The figure shows three views and two pictorial views of one solid part (mm, origin at its lowest corner). Answer the questions. A direction names the side the tool comes from. Coordinates: 2 decimals unless noted, no trailing zeros. Loops run counter-clockwise (first coordinate to the right, second up) from the corner with the lowest first, then second, coordinate; pieces in that order, holes last. Notation, with made-up numbers: M 2,67 L 59,67 A8 cw 59,76 Z; hole C -16.5,69 d9. An arc over 180 degrees is marked long. One line per item, written item: value. Start each with the question number.
1. The part is cut by section B-B (y = 2.54). Write down the section's boundary in (x, z), then the cut area to 3 significant figures.
2. The part is cut by section A-A (y = 4.75). Write down the section's boundary in (x, z).
3. A flat-ended cylindrical pin translates along its axis: pin 1 (3 mm diameter, centred on x = 8, z = 4, fed in from -Y). Find the tip coordinate at first contact, or state that the pin passes through.
4. For the marked faces 1 and 2, determine the directions among +Z, -Z, +X, -X, +Y, -Y from which every point of the face is accessible in a straight line to the end or side of a thin tool.
5. Consider probe 1 along X at (y, z) = (3.75, 9.25); probe 2 along Y at (x, z) = (1.3, 5.08); probe 3 along Y at (x, z) = (19.75, 3.25). Determine where each line is inside the solid, lowest interval first.
6. Determine the mould class of the marked faces 3, 4 and 5 for opening direction X: +X half, -X half, draft (parallel to the pull), parting line (faces both ways), or undercut.
7. The part is cut by section D-D (x = 12.7). Write down the section's boundary in (y, z), then the cut area to 3 significant figures.
8. The part is cut by section C-C (z = 5.08). Write down the section's boundary in (x, y).
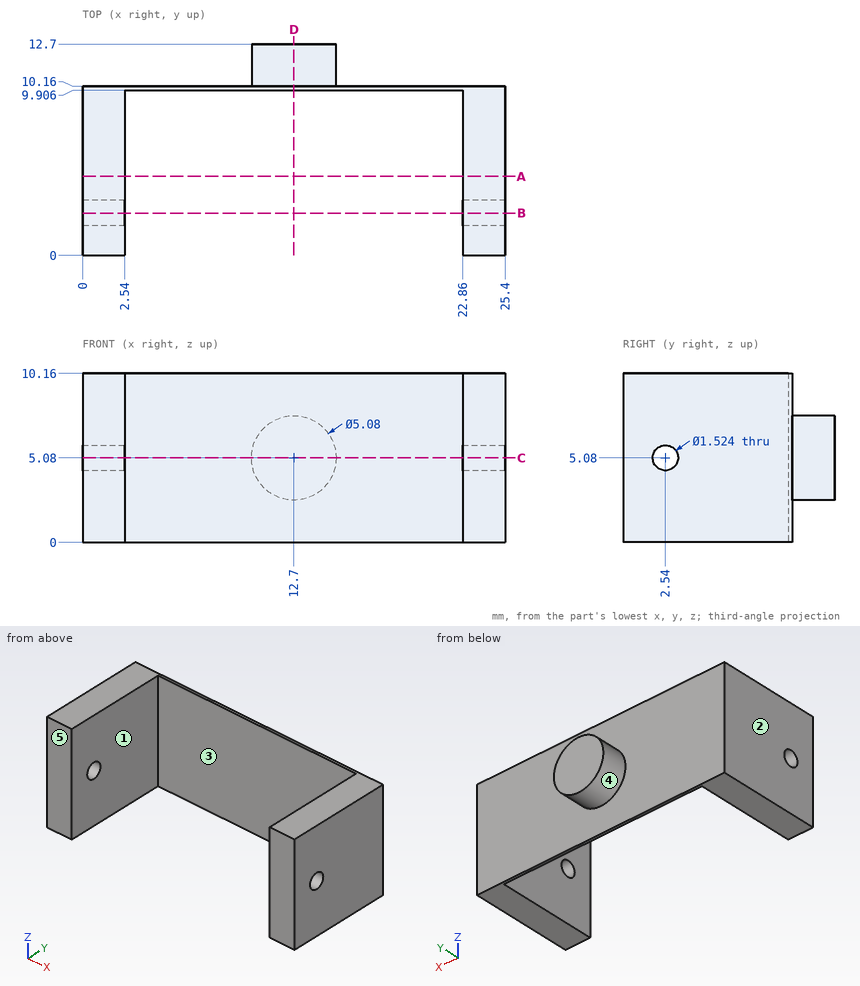
Answer block:
1. outline: M 0,0 L 2.54,0 L 2.54,4.32 L 0,4.32 Z; M 0,5.84 L 2.54,5.84 L 2.54,10.16 L 0,10.16 Z; M 22.86,0 L 25.4,0 L 25.4,4.32 L 22.86,4.32 Z; M 22.86,5.84 L 25.4,5.84 L 25.4,10.16 L 22.86,10.16 Z
1. area: 43.9 mm2
2. outline: M 0,0 L 2.54,0 L 2.54,10.16 L 0,10.16 Z; M 22.86,0 L 25.4,0 L 25.4,10.16 L 22.86,10.16 Z
3. pin 1: stops at y = 9.91
4. face 1: +Z, -Z, -Y
4. face 2: +Z, -Z, -X, +Y, -Y
5. probe 1: x = 0 to 2.54, 22.86 to 25.4
5. probe 2: y = 0 to 1.78, 3.3 to 10.16
5. probe 3: y = 9.91 to 10.16
6. face 3: undercut
6. face 4: parting line
6. face 5: draft
7. outline: M 9.91,0 L 10.16,0 L 10.16,2.54 L 12.7,2.54 L 12.7,7.62 L 10.16,7.62 L 10.16,10.16 L 9.91,10.16 Z
7. area: 15.5 mm2
8. outline: M 0,0 L 2.54,0 L 2.54,1.78 L 0,1.78 Z; M 0,3.3 L 2.54,3.3 L 2.54,9.91 L 22.86,9.91 L 22.86,3.3 L 25.4,3.3 L 25.4,10.16 L 15.24,10.16 L 15.24,12.7 L 10.16,12.7 L 10.16,10.16 L 0,10.16 Z; M 22.86,0 L 25.4,0 L 25.4,1.78 L 22.86,1.78 Z
